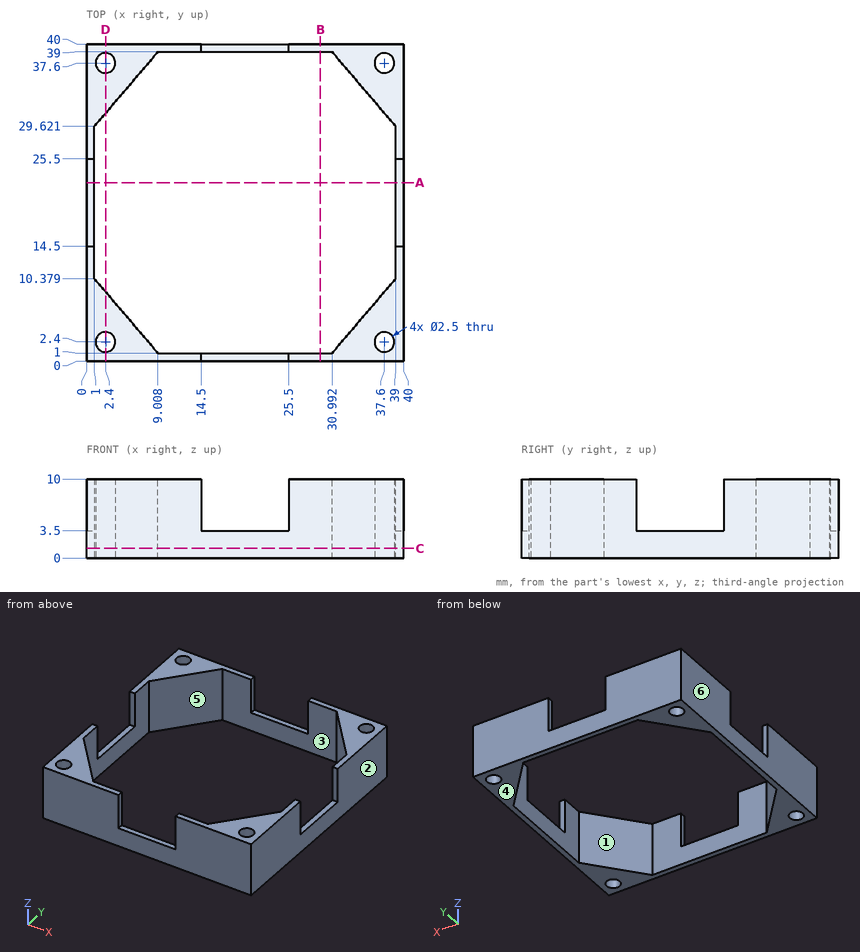
Input: dimensioned drawing with shaded views. Units: mm. Origin: part minimum x, y, z. A direction names the side the tool comes from. Give positions to 0.01 mm unless a question says otherwise; leave off trailing zeros. Loops run counter-clockwise (first coordinate to the right, second up) from the corner with the lowest first, then second, coordinate; pieces in that order, holes last. Notation, with made-up numbers: (31, 75.5) - (40, 75.5) arc R12 ccw to (40, 90.5) - close; hole circle Ø4 at (-30.5, 85.5). An arc over 180 degrees is marked (long way). Answer as CSV lines item,"result". Start each with the question number.
(1) Section query B-B (x = 29.5). Output: boundary loops of the cut face in (y, z).
(2) Section query C-C (z = 1.25). Output: boundary loops of the cut face in (x, y).
(3) Ray query, line 1 along X through (y, z) = (26, 5); line 2 along Y through (x, z) = (37.6, 6.75). Return the intervals inside material, ascending. Write a range as [from, to].
(4) Section query D-D (x = 2.4). Output: boundary loops of the cut face in (y, z), and give its area (3 significant figures).
(5) Pin query (flat end, axial travel): P1, Ø1.1, axis at x = 39.5, y = 22.5, coming from the +Z side. Return the tip coordinate at first contact, or that it passes through.
(6) Reachability of the marked faces 1 and 2 from +Z, -Z, +X, -X, +Y, -Y: full face, straight path, thin tool, end or side. Return the list, or none.
(7) Mould query, pull axis X, two halves, no side actions, for the marked faces 3, 4, 5 and 6. Classes: +X half, -X half, draft (parallel to the pull), parting line (faces both ways), or undercut.
(8) Section query A-A (y = 22.5). Output: boundary loops of the cut face in (x, z).
Worked answers:
1,outline,"(0, 0) - (1, 0) - (1, 10) - (0, 10) - close; (39, 0) - (40, 0) - (40, 10) - (39, 10) - close"
2,outline,"(0, 0) - (40, 0) - (40, 40) - (0, 40) - close; hole (1, 10.38) - (9.01, 1) - (30.99, 1) - (39, 10.38) - (39, 29.62) - (30.99, 39) - (9.01, 39) - (1, 29.62) - close; hole circle Ø2.5 at (2.4, 2.4); hole circle Ø2.5 at (2.4, 37.6); hole circle Ø2.5 at (37.6, 2.4); hole circle Ø2.5 at (37.6, 37.6)"
3,line 1,"x = [0, 1], [39, 40]"
3,line 2,"y = [0, 1.15], [3.65, 8.74], [31.26, 36.35], [38.85, 40]"
4,outline,"(0, 0) - (1.15, 0) - (1.15, 10) - (0, 10) - close; (3.65, 0) - (8.74, 0) - (8.74, 10) - (3.65, 10) - close; (31.26, 0) - (36.35, 0) - (36.35, 10) - (31.26, 10) - close; (38.85, 0) - (40, 0) - (40, 10) - (38.85, 10) - close"
4,area,"125 mm^2"
5,P1,"stops at z = 3.5"
6,face 1,"+Z, -Z"
6,face 2,"+Z, -Z, +X, +Y, -Y"
7,face 3,"undercut"
7,face 4,"draft"
7,face 5,"undercut"
7,face 6,"-X half"
8,outline,"(0, 0) - (1, 0) - (1, 3.5) - (0, 3.5) - close; (39, 0) - (40, 0) - (40, 3.5) - (39, 3.5) - close"
